```python
from build123d import *

# Parameters (mm, degrees)
SKIZZE1_W                       = 20
SKIZZE1_H                       = 40
AUFSATZ_LINEAR_AUSTRAGEN1_DEPTH = 4


with BuildPart() as part:
    # Skizze1 → Aufsatz-Linear austragen1 (new body)
    with BuildSketch(Plane.XY):
        Polygon((0, 0), (80, 0), (80, 6), (110, 6), (110, 0), (125, 0), (125, 110), (25, 110), (25, 75), (0, 75), align=None)
        with Locations((107, 80)):
            Rectangle(SKIZZE1_W, SKIZZE1_H, mode=Mode.SUBTRACT)
    extrude(amount=AUFSATZ_LINEAR_AUSTRAGEN1_DEPTH)


solid = part.part
```
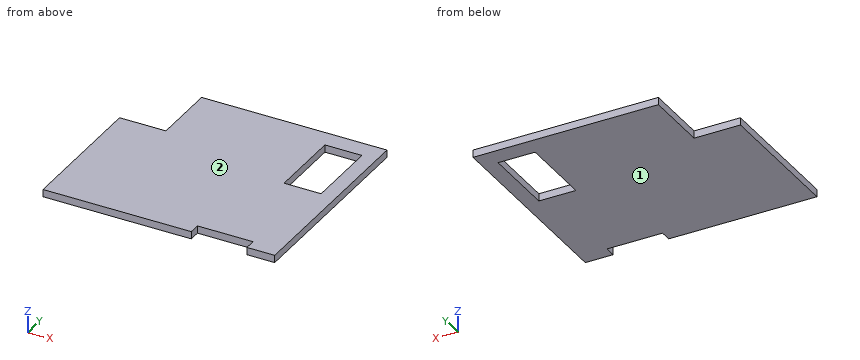
Build history of the part. All positions in model axes, mm. Face numbers are marked on the shaded views. Round coordinates to 2 decimals unless told otherwise and drop trailing zeros. Write each loop counter-clockwise with the first axis right and the second up, starting at its lowest first coordinate (ties: lowest second). Pieces come first, ordered by that corner, then holes. Notation, with made-up numbers: (-34, -10) - (11, -10) arc R21 ccw to (11, 7) - close; hole circle Ø10 at (3.25, 70). An arc over 180 degrees is marked (long way). Write each question's results on one line, items separated by ' | '. Start each with the question number.
Item 1: Saw through at A-A (y = 73). Write the cut outline in (x, z).
Item 2: Drop a flat-ended pin along its axis: P1, Ø1.2, axis at x = 108.5, z = 1, coming from the -Y side. Give the stop position or say it passes through.
Item 3: Saw through at C-C (x = 93.5). Write the cut outline in (y, z).
Item 4: Mould opens along Z. For the marked faces 1 and 2 say: pulls with the +Z half, pulls with the -Z half, needs draft (parallel to the pull), parting line crosses it, or undercut.
Item 5: Wall check: L1, parallel to X at y = 88, z = 1.6; L2, parallel to X at y = 71, z = 2.5; L3, parallel to Y at x = 84, z = 2.9. Give the ranges that are in metal, low to high. Write a range as [from, to].
Item 6: Saw through at B-B (z = 3.4). Write the cut outline in (x, y), and give its area (3 significant figures).
Results are:
1) outline: (0, 0) - (97, 0) - (97, 4) - (0, 4) - close; (117, 0) - (125, 0) - (125, 4) - (117, 4) - close
2) P1: stops at y = 6
3) outline: (6, 0) - (110, 0) - (110, 4) - (6, 4) - close
4) face 1: pulls with the -Z half | face 2: pulls with the +Z half
5) L1: x = [25, 97], [117, 125] | L2: x = [0, 97], [117, 125] | L3: y = [6, 110]
6) outline: (0, 0) - (80, 0) - (80, 6) - (110, 6) - (110, 0) - (125, 0) - (125, 110) - (25, 110) - (25, 75) - (0, 75) - close; hole (97, 60) - (117, 60) - (117, 100) - (97, 100) - close | area: 11,900 mm²
